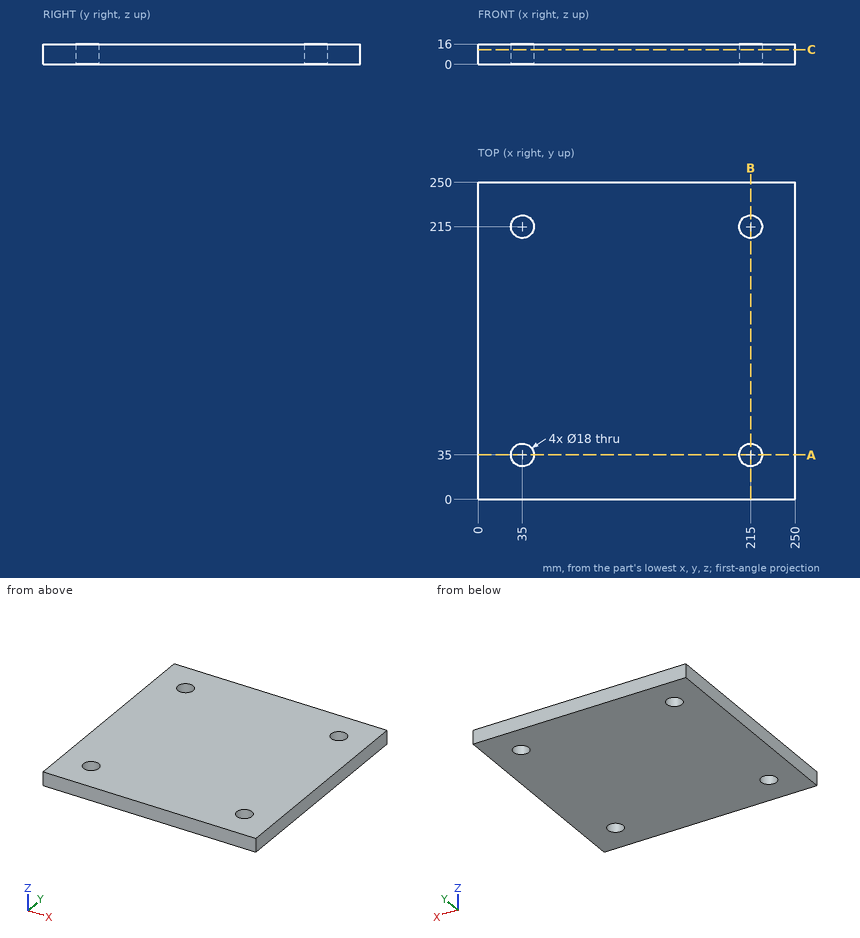
For this review, use the dimensioned drawing (mm, ordinates from the lowest corner) and the shaded views. Give positions to 0.01 mm unless a question says otherwise; leave off trailing zeros. Write each loop counter-clockwise with the first axis right and the second up, starting at its lowest first coordinate (ties: lowest second). Pieces come first, ordered by that corner, then holes.
(1) For P1, Ø14.5, axis at x = 35, y = 215, coming from the +Z side, flat-tipped, find the tip position at first contact; note if it passes through.
(2) To check wall thickness, follow L1, parallel to Y at x = 215, z = 4.5; L2, parallel to X at y = 216.5, z = 2.5; L3, parallel to Y at x = 41.5, z = 11.75. State the ranges of each line that lie inside material, in increasing order.
(3) Consider section A-A, the plane y = 35. Give the boundary of the cut face in (x, z), and give its area (3 significant figures).
(4) Consider section C-C, the plane z = 11.5. Give the boundary of the cut face in (x, y), and give its area (3 significant figures).
Returned:
1. P1: passes through
2. L1: y = 0 to 26, 44 to 206, 224 to 250
2. L2: x = 0 to 26.13, 43.87 to 206.13, 223.87 to 250
2. L3: y = 0 to 28.78, 41.22 to 208.78, 221.22 to 250
3. outline: (0, 0) - (26, 0) - (26, 16) - (0, 16) - close; (44, 0) - (206, 0) - (206, 16) - (44, 16) - close; (224, 0) - (250, 0) - (250, 16) - (224, 16) - close
3. area: 3,420 mm2
4. outline: (0, 0) - (250, 0) - (250, 250) - (0, 250) - close; hole circle Ø18 at (35, 35); hole circle Ø18 at (35, 215); hole circle Ø18 at (215, 35); hole circle Ø18 at (215, 215)
4. area: 61,500 mm2
